from build123d import *
from build123d import SkipClean  # not in build123d's __all__

# Parameters (mm, degrees)
F2_W     = 200
F2_H     = 100
F2_H_2   = 20
F3_DEPTH = 100
F2_W_2   = 75
F2_H_3   = 25
F6_DEPTH = 35
F8_W     = 96.0638802499
F8_H     = 5.2582259355
F9_DEPTH = 50


# Not quite as in the source:
# - ends of sketch curves that miss each other by under 0.0002 mm in the source are joined
# - a feature of the source that left no trace in its solid (it failed there, or was rolled back) is left out
# - a feature names something its author has since deleted; it is built from what else it names


with BuildPart() as f1:
    # F0 (on Front) → F1 (revolve)
    with BuildSketch(Plane.XZ):
        with BuildLine():
            add(Edge.make_bspline(
                [(45.9368361786, 26.8256458213), (91.5796084466, 124.7068868213), (26.32544778, 155.1354016666)],
                knots=[4.7123889804, 4.7123889804, 4.7123889804, 6.2831853072, 6.2831853072, 6.2831853072], degree=2, weights=[1, 0.7071067812, 1]))
            Line((26.32544778, 155.1354016666), (25.4802112565, 153.3227860925))
            add(Edge.make_bspline(
                [(44.1242206045, 27.6708823448), (88.921756349, 123.7395077707), (25.4802112565, 153.3227860925)],
                knots=[4.7123889804, 4.7123889804, 4.7123889804, 6.2831853072, 6.2831853072, 6.2831853072], degree=2, weights=[1, 0.7071067812, 1]))
            Line((44.1242206045, 27.6708823448), (45.9368361786, 26.8256458213))
        make_face()
    revolve(axis=Axis((-11.7101957767, 0, 73.5677008333), (-0.4226182617, 0, -0.906307787)))


with BuildPart() as f1b:
    # F0 (on Front) → F1, piece 2 (revolve)
    with BuildSketch(Plane.XZ):
        Polygon((0.1731735164, 31.6149234015), (-1.1862881642, 32.2488507941), (-15.9779273251, 0.5280782478), (-14.6184656445, -0.1058491448), align=None)
        with BuildLine():
            add(Edge.make_bspline(
                [(-22.1410875874, -12.6888615869), (-21.3247514691, -12.7218189818), (-20.5078685114, -12.7357143506)],
                knots=[0.3959818916, 0.3959818916, 0.3959818916, 0.4193237212, 0.4193237212, 0.4193237212], degree=2, weights=[1, 0.9999318956, 1]))
            Line((-20.5078685114, -12.7357143506), (-14.6184656445, -0.1058491448))
            Line((-14.6184656445, -0.1058491448), (-15.9779273251, 0.5280782478))
            Line((-15.9779273251, 0.5280782478), (-22.1410875874, -12.6888615869))
        make_face()
    revolve(axis=Axis((-11.7101957767, 0, 73.5677008333), (-0.4226182617, 0, -0.906307787)))


with BuildPart() as f3_tool:
    # F2 (on Front) → F3 (new body, symmetric)
    with BuildSketch(Plane.XZ):
        with Locations((-9.317324488, 115)):
            Rectangle(F2_W, F2_H)
        with Locations((0, -10)):
            Rectangle(F2_W, F2_H_2)
    extrude(amount=F3_DEPTH, both=True)


with BuildPart() as f1_1:
    add(f1.part, clean=False)

    # F3: cut by f3_tool
    add(f3_tool.part, mode=Mode.SUBTRACT)

    # F0 (on Front) → F7 (revolve, cut)
    with BuildSketch(Plane.XZ):
        with BuildLine():
            add(Edge.make_bspline(
                [(-84.5714851547, 87.682675512), (-114.9949652888, 22.4393118183), (-49.756636783, -7.9949639789)],
                knots=[4.7123889804, 4.7123889804, 4.7123889804, 6.2830198332, 6.2830198332, 6.2830198332], degree=2, weights=[1, 0.7071652827, 1]))
            Line((-49.756636783, -7.9949639789), (-49.7458393334, -8))
            Line((-49.7458393334, -8), (-49.735042102, -8.0050348317))
            add(Edge.make_bspline(
                [(-49.735042102, -8.0050348317), (15.5133557484, -38.4177185072), (45.9368361786, 26.8256458213)],
                knots=[0.0001654643, 0.0001654643, 0.0001654643, 1.5707963268, 1.5707963268, 1.5707963268], degree=2, weights=[1, 0.7071652792, 1]))
            Line((45.9368361786, 26.8256458213), (44.1242206045, 27.6708823448))
            add(Edge.make_bspline(
                [(-20.5078685114, -12.7357143506), (24.9219656119, -13.5084863764), (44.1242206045, 27.6708823448)],
                knots=[0.4193237212, 0.4193237212, 0.4193237212, 1.5707963268, 1.5707963268, 1.5707963268], degree=2, weights=[1, 0.8387916479, 1]))
            add(Edge.make_bspline(
                [(-22.1410875874, -12.6888615869), (-21.3247514691, -12.7218189818), (-20.5078685114, -12.7357143506)],
                knots=[0.3959818916, 0.3959818916, 0.3959818916, 0.4193237212, 0.4193237212, 0.4193237212], degree=2, weights=[1, 0.9999318956, 1]))
            add(Edge.make_bspline(
                [(-38.8967253804, -9.951843981), (-30.686098613, -12.3438795424), (-22.1410875874, -12.6888615869)],
                knots=[0.1528447244, 0.1528447244, 0.1528447244, 0.3959818916, 0.3959818916, 0.3959818916], degree=2, weights=[1, 0.9926196359, 1]))
            add(Edge.make_bspline(
                [(-48.9006028099, -6.1873844259), (-44.042789232, -8.4526200992), (-38.8967253804, -9.951843981)],
                knots=[0, 0, 0, 0.1528447244, 0.1528447244, 0.1528447244], degree=2, weights=[1, 0.9970812323, 1]))
            add(Edge.make_bspline(
                [(-48.9112500264, -6.1824184595), (-48.9059266265, -6.1849018895), (-48.9006028099, -6.1873844259)],
                knots=[6.2830174734, 6.2830174734, 6.2830174734, 6.2831853072, 6.2831853072, 6.2831853072], degree=2, weights=[1, 0.9999999965, 1]))
            add(Edge.make_bspline(
                [(-71.0817080874, 10.1325245471), (-61.6323129878, -0.2478899078), (-48.9112500264, -6.1824184595)],
                knots=[5.8872034156, 5.8872034156, 5.8872034156, 6.2830174734, 6.2830174734, 6.2830174734], degree=2, weights=[1, 0.9804802401, 1]))
            add(Edge.make_bspline(
                [(-72.1674123725, 11.3535265686), (-71.6316856587, 10.7366896891), (-71.0817080874, 10.1325245471)],
                knots=[5.863861586, 5.863861586, 5.863861586, 5.8872034156, 5.8872034156, 5.8872034156], degree=2, weights=[1, 0.9999318956, 1]))
            add(Edge.make_bspline(
                [(-82.7588695806, 86.8374389885), (-101.9611245733, 45.6580702673), (-72.1674123725, 11.3535265686)],
                knots=[4.7123889804, 4.7123889804, 4.7123889804, 5.863861586, 5.863861586, 5.863861586], degree=2, weights=[1, 0.8387916479, 1]))
            Line((-82.7588695806, 86.8374389885), (-84.5714851547, 87.682675512))
        make_face()
        with BuildLine():
            add(Edge.make_bspline(
                [(26.32544778, 155.1354016666), (-38.9287128867, 185.5639165119), (-84.5714851547, 87.682675512)],
                knots=[0, 0, 0, 1.5707963268, 1.5707963268, 1.5707963268], degree=2, weights=[1, 0.7071067812, 1]))
            Line((-84.5714851547, 87.682675512), (-82.7588695806, 86.8374389885))
            add(Edge.make_bspline(
                [(25.4802112565, 153.3227860925), (-37.9613338361, 182.9060644144), (-82.7588695806, 86.8374389885)],
                knots=[0, 0, 0, 1.5707963268, 1.5707963268, 1.5707963268], degree=2, weights=[1, 0.7071067812, 1]))
            Line((25.4802112565, 153.3227860925), (26.32544778, 155.1354016666))
        make_face()
    with SkipClean():  # cleaning this boolean's faces spoils the solid; the shape is the same uncleaned
        revolve(axis=Axis((-11.7101957767, 0, 73.5677008333), (-0.4226182617, 0, -0.906307787)), mode=Mode.SUBTRACT)


with BuildPart() as f1b_1:
    add(f1b.part, clean=False)

    # F3: cut by f3_tool
    add(f3_tool.part, mode=Mode.SUBTRACT)

    # F2 (on Front) → F6 (cut, symmetric)
    with BuildSketch(Plane.XZ):
        with Locations((-37.3268264836, 44.1149234015)):
            Rectangle(F2_W_2, F2_H_3)
    extrude(amount=F6_DEPTH, both=True, mode=Mode.SUBTRACT)

    # F8 (on Front) → F9 (cut, symmetric)
    with BuildSketch(Plane.XZ):
        with Locations((-19.0352806821, -1.4191129678)):
            Rectangle(F8_W, F8_H)
    extrude(amount=F9_DEPTH, both=True, mode=Mode.SUBTRACT)


solid = f1b_1.part
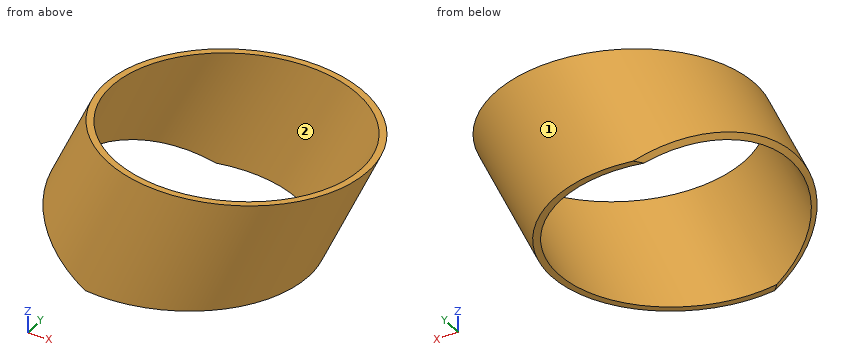
Can you work these out from the model? Positions are in its coordinate system, mm. Face numbers are marked on the shaded views. Give positions to 0.01 mm unless a question says otherwise; leave off trailing zeros. Return JSON: item names as keys, results as strings.
Q1. For pin 1 Ø1.5 at (y, z) = (11.5, 20.5) entering from -X; pin 2 Ø6 at (x, y) = (-55, 14) entering from +Z; pin 3 Ø1 at (y, z) = (5, 23.5) entering from +X; pin 4 Ø1 at (x, z) = (-41.5, 6) entering from -Y, each with a flat end and sliding along its axis, tell me the tip position at first contact or that it passes through.
Checks:
{"pin 1": "stops at x = -65.73", "pin 2": "stops at z = 31.61", "pin 3": "stops at x = -3.85", "pin 4": "stops at y = -28.48"}
Q2. I need wall thicknesses on probe 1 along Y at (x, z) = (-59, 14.5); probe 2 along X at (y, z) = (23, 19); probe 3 along Y at (x, z) = (-63.5, 19.5). Which ranges of each line are inside material? Lowest first, please.
Checks:
{"probe 1": "y = -22.18 to -20.22, 20.22 to 22.18", "probe 2": "x = -55.73 to -52.76, -21.55 to -18.59", "probe 3": "y = -15.23 to -12.2, 12.2 to 15.23"}
Q3. We'd pull the mould along Y, two halves only. Please class the marked faces 1 and 2: released by +Y, released by -Y, zero draft, split by the parting line, or undercut.
Checks:
{"face 1": "split by the parting line", "face 2": "undercut"}
